Can you work these out from the model? Positions are in its coordinate system, mm. A direction names the side the tool comes from. Round coordinates to 2 decimals unless told otherwise and drop trailing zeros. Loops run counter-clockwise (first coordinate to the right, second up) from the corner with the lowest first, then second, coordinate; pieces in that order, holes last. Notation, with made-up numbers: (-1.75, -2) -> (55.25, -2) arc R13 ccw to (55.25, 18) -> close; hole circle Ø6 at (83.5, -0.5). An arc over 180 degrees is marked (long way). Write item = value, one per line.
from build123d import *

# Parameters (mm, degrees)
SKETCH_1_W                       = 102
SKETCH_1_H                       = 80
SKETCH_1_R                       = 1.6
EXTRUDE_1_DEPTH                  = 3
CUT_EXTRUDE_1_DEPTH              = 3
SKETCH_4_W                       = 5.1
SKETCH_4_H                       = 5.5
CUT_EXTRUDE_2_DEPTH              = 5
PATTERN_LINEAR_1_COUNT           = 2
PATTERN_LINEAR_1_PITCH           = 62.5
PATTERN_LINEAR_1_COPY_1_SKETCH_W = 5.1
PATTERN_LINEAR_1_COPY_1_SKETCH_H = 5.5
PATTERN_LINEAR_1_COPY_1_DEPTH    = 5


with BuildPart() as part:
    # 草图1 → 凸台-拉伸1 (new body)
    with BuildSketch(Plane.XY):
        with Locations((0, -65.25)):
            Rectangle(SKETCH_1_W, SKETCH_1_H)
        with Locations((-38, -35.25)):
            Circle(SKETCH_1_R, mode=Mode.SUBTRACT)
        with Locations((-38, -95.25)):
            Circle(SKETCH_1_R, mode=Mode.SUBTRACT)
        with Locations((38, -95.25)):
            Circle(SKETCH_1_R, mode=Mode.SUBTRACT)
        with Locations((38, -35.25)):
            Circle(SKETCH_1_R, mode=Mode.SUBTRACT)
    extrude(amount=EXTRUDE_1_DEPTH)

    # 草图3 → 切除-拉伸1 (cut)
    with BuildSketch(Plane.XY.offset(3)):
        with BuildLine():
            Line((-2.065542075, -33.415194888), (4.318378476, -33.415194888))
            ThreePointArc((4.318378476, -33.415194888), (8.318378476, -37.415194888), (4.318378476, -41.415194888))
            Line((4.318378476, -41.415194888), (-2.065542075, -41.415194888))
            ThreePointArc((-2.065542075, -41.415194888), (-6.065542075, -37.415194888), (-2.065542075, -33.415194888))
        make_face()
    extrude(amount=-CUT_EXTRUDE_1_DEPTH, mode=Mode.SUBTRACT)

    # 草图4 → 切除-拉伸2 (cut)
    with BuildSketch(Plane.XY.offset(3)):
        with Locations((-24.95, -97.5)):
            Rectangle(SKETCH_4_W, SKETCH_4_H)
    cut_extrude_2 = extrude(amount=-CUT_EXTRUDE_2_DEPTH, mode=Mode.SUBTRACT)

    # 镜向1: 切除-拉伸2 across plane
    add(cut_extrude_2.mirror(Plane.ZY), mode=Mode.SUBTRACT)

    # 阵列(线性)1: 切除-拉伸2 ×2
    with Locations(*[(0, i * PATTERN_LINEAR_1_PITCH, 0) for i in range(1, PATTERN_LINEAR_1_COUNT)]):
        add(cut_extrude_2, mode=Mode.SUBTRACT)

    # 阵列(线性)1 copy 1 sketch → 阵列(线性)1 copy 1 (cut)
    with BuildSketch(Plane(origin=(0, 62.5, 3), x_dir=(-1, 0, 0), z_dir=(0, 0, 1))):
        with Locations((-24.95, 97.5)):
            Rectangle(PATTERN_LINEAR_1_COPY_1_SKETCH_W, PATTERN_LINEAR_1_COPY_1_SKETCH_H)
    extrude(amount=-PATTERN_LINEAR_1_COPY_1_DEPTH, mode=Mode.SUBTRACT)


solid = part.part
1. I'm going to push a flat-ended pin straight in: pin 1 (3 mm diameter, centred on x = -38, y = -95.25, fed in from +Z). Where does the tip first touch, or does it pass through?
Entries:
pin_1 = through
2. Suppose I cut it at D-D, the plane x = 26. List the corners of the cut face in (y, z) for me, and give its area (3 significant figures).
Entries:
outline = (-105.25, 0) -> (-100.25, 0) -> (-100.25, 3) -> (-105.25, 3) -> close; (-94.75, 0) -> (-37.75, 0) -> (-37.75, 3) -> (-94.75, 3) -> close; (-32.25, 0) -> (-25.25, 0) -> (-25.25, 3) -> (-32.25, 3) -> close
area = 207 mm²
3. For faces 1 (the flat face through (-1, -65, 3)), 2 (the flat face through (1, -41.415, 2)), which set-ups out of +Z, -Z, +X, -X, +Y, -Y let a thin tool reach every point of the face, with its end or its side?
Entries:
face_1 = +Z, +X, -X, +Y, -Y
face_2 = +Z, -Z
4. Suppose I cut it at B-B, the plane z = 0.55. Count the separate pieces of the cut face and the enclosed holes in it, and give its area (3 significant figures).
Entries:
separate_pieces = 1
enclosed_holes = 9
area = 7,910 mm²
5. Suppose I cut it at A-A, the plane x = 38. List the corners of the cut face in (y, z) for me.
Entries:
outline = (-105.25, 0) -> (-96.85, 0) -> (-96.85, 3) -> (-105.25, 3) -> close; (-93.65, 0) -> (-36.85, 0) -> (-36.85, 3) -> (-93.65, 3) -> close; (-33.65, 0) -> (-25.25, 0) -> (-25.25, 3) -> (-33.65, 3) -> close
6. I need wall thicknesses on line 1 (Y direction, x = -38, z = 1.4); line 2 (X direction, y = -95.25, z = 0.85); line 3 (Y direction, x = 4, z = 1.8). Which ranges of each line are inside material? Lowest first, please. Write a range as [from, to].
Entries:
line_1 = [-105.25, -96.85], [-93.65, -36.85], [-33.65, -25.25]
line_2 = [-51, -39.6], [-36.4, -27.5], [-22.4, 22.4], [27.5, 36.4], [39.6, 51]
line_3 = [-105.25, -41.42], [-33.42, -25.25]
7. Suppose I cut it at C-C, the plane y = -35.25. List the corners of the cut face in (x, z) for me, and give its area (3 significant figures).
Entries:
outline = (-51, 0) -> (-39.6, 0) -> (-39.6, 3) -> (-51, 3) -> close; (-36.4, 0) -> (-27.5, 0) -> (-27.5, 3) -> (-36.4, 3) -> close; (-22.4, 0) -> (-5.43, 0) -> (-5.43, 3) -> (-22.4, 3) -> close; (7.68, 0) -> (22.4, 0) -> (22.4, 3) -> (7.68, 3) -> close; (27.5, 0) -> (36.4, 0) -> (36.4, 3) -> (27.5, 3) -> close; (39.6, 0) -> (51, 0) -> (51, 3) -> (39.6, 3) -> close
area = 217 mm²
